Source: three-view drawing plus pictorial views. Frame: mm from the lowest corner of the part. A direction names the side the tool comes from. Give positions to 0.01 mm unless a question says otherwise; leave off trailing zeros. Order: outer loops, then holes, each group sorted by start corner. A loop starts at its lowest first (then second) coordinate and runs counter-clockwise, first axis right, second up. Notation, with made-up numbers: M 59,80.25 L 76,80.25 A26 ccw 76,101.25 Z; hole C -9.5,-3 d4. An arc over 180 degrees is marked long. Use CSV: the item, a comma, the result in double quotes. Start each with the question number.
Item 1: Section query C-C on z = 61. Return loops of the section in (x, y).
Item 2: Section query D-D on y = 152. Return loops of the section in (x, z).
Item 3: Section query B-B on x = 77. Return loops of the section in (y, z), and give its area (3 significant figures).
Item 4: Access query for the marked faces 1, 2 and 3. Directions: +Z, -Z, +X, -X, +Y, -Y. A direction counts if a zero-diameter tool reaches every point of the face in a straight line with its end or side. Return the directions, or none.
Item 5: First-contact query: pin 1 (5 mm diameter, centred on x = 64.5, y = 65.5, fed in from +Z); pin 2 (4 mm diameter, centred on x = 172.5, y = 151.5, fed in from +Z); pin 3 (3 mm diameter, centred on x = 85.5, z = 83.5, fed in from +Y); pin 4 (6 mm diameter, centred on x = 92, z = 29.5, fed in from +Y). Flat tips, straight axial feed; report the tip coordinate or a pass-through.
Item 6: Ray query, probe 1 along Z at (x, y) = (34.5, 190); probe 2 along Y at (x, z) = (46, 29); probe 3 along Z at (x, y) = (148, 91.5). Return the intervals inside material, ascending. Write a range as from..to.
Item 7: Section query A-A on y = 82. Return loops of the section in (x, z), and give its area (3 significant figures).
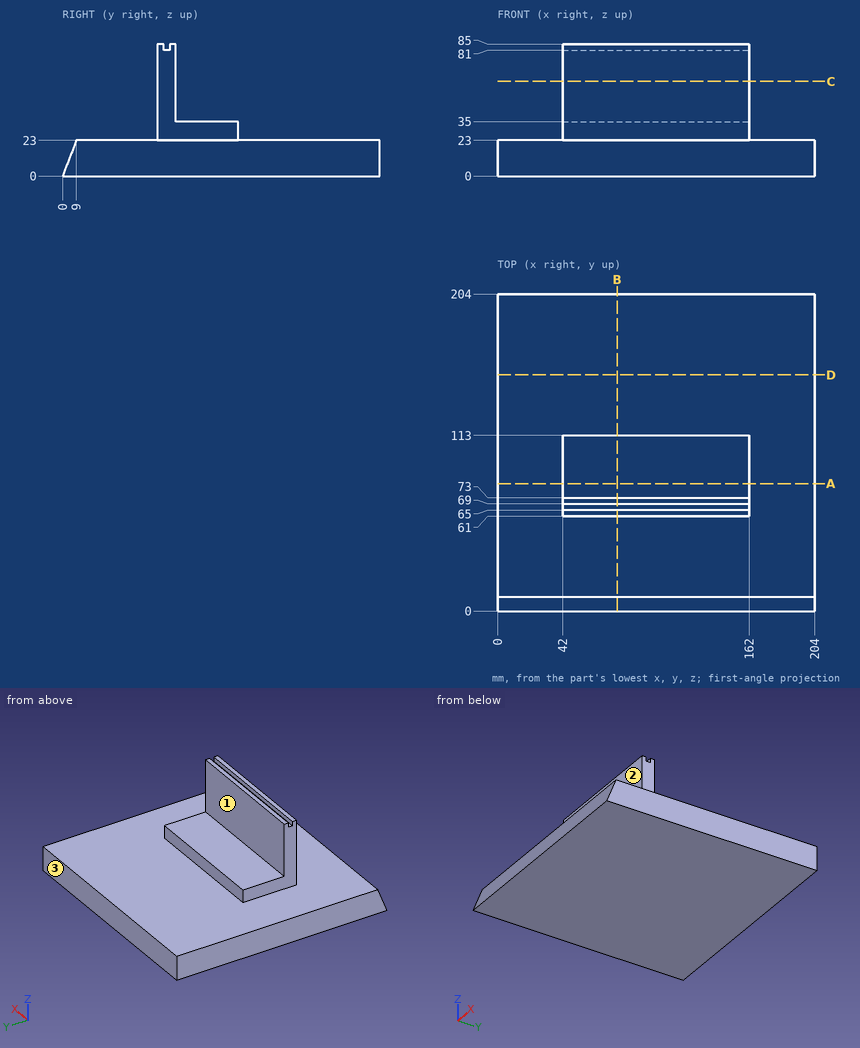
Verdict:
1,outline,"M 42,61 L 162,61 L 162,73 L 42,73 Z"
2,outline,"M 0,0 L 204,0 L 204,23 L 0,23 Z"
3,outline,"M 0,0 L 204,0 L 204,23 L 113,23 L 113,35 L 73,35 L 73,85 L 69,85 L 69,81 L 65,81 L 65,85 L 61,85 L 61,23 L 9,23 Z"
3,area,"5,800 mm2"
4,face 1,"+Z, +X, -X, +Y"
4,face 2,"+Z, +X, -X, -Y"
4,face 3,"+Z, -Z, +X, -X, +Y"
5,pin 1,"z = 85"
5,pin 2,"z = 23"
5,pin 3,"y = 73"
5,pin 4,"y = 113"
6,probe 1,"0..23"
6,probe 2,"61..113"
6,probe 3,"0..35"
7,outline,"M 0,0 L 204,0 L 204,23 L 162,23 L 162,35 L 42,35 L 42,23 L 0,23 Z"
7,area,"6,130 mm2"
